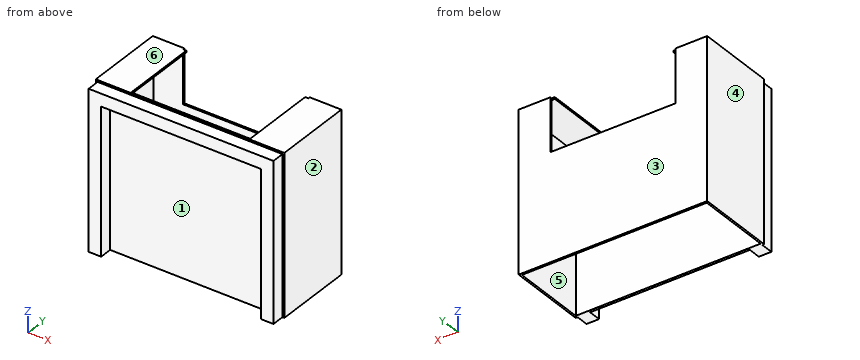
from build123d import *

# Parameters (mm, degrees)
SKETCH_1_W          = 602.574462866
SKETCH_1_H          = 504.761774505
EXTRUDE_1_DEPTH     = 8
SKETCH_2_W          = 6
SKETCH_2_H          = 504.761774505
EXTRUDE_2_DEPTH     = 240
SKETCH_3_W          = 602.574462866
SKETCH_3_H          = 504.761774505
EXTRUDE_3_DEPTH     = 6
SKETCH_5_W          = 602.574462866
SKETCH_5_H          = 254
EXTRUDE_4_DEPTH     = 6
SKETCH_4_W          = 400
SKETCH_4_H          = 170
CUT_EXTRUDE_4_DEPTH = 6
SKETCH_9_W          = 380
SKETCH_9_H          = 245
CUT_EXTRUDE_5_DEPTH = 6
EXTRUDE_8_DEPTH     = 40


with BuildPart() as part:
    # Эскиз1 → Бобышка-Вытянуть1 (new body)
    with BuildSketch(Plane(origin=(0, 0, 0), x_dir=(1, 0, 0), z_dir=(0, 1, 0))):
        with Locations((300, -321.529892077)):
            Rectangle(SKETCH_1_W, SKETCH_1_H)
    extrude(amount=EXTRUDE_1_DEPTH)

    # Эскиз2 → Бобышка-Вытянуть2 (add)
    with BuildSketch(Plane(origin=(0, 8, 0), x_dir=(1, 0, 0), z_dir=(0, 1, 0))):
        with Locations((1.712768567, -321.529892077)):
            Rectangle(SKETCH_2_W, SKETCH_2_H)
        with Locations((598.287231433, -321.529892077)):
            Rectangle(SKETCH_2_W, SKETCH_2_H)
    extrude(amount=EXTRUDE_2_DEPTH)

    # Эскиз3 → Бобышка-Вытянуть3 (add)
    with BuildSketch(Plane(origin=(0, 248, 0), x_dir=(1, 0, 0), z_dir=(0, 1, 0))):
        with Locations((300, -321.529892077)):
            Rectangle(SKETCH_3_W, SKETCH_3_H)
    extrude(amount=EXTRUDE_3_DEPTH)

    # Эскиз5 → Бобышка-Вытянуть4 (add)
    with BuildSketch(Plane.XY.offset(573.910779329)):
        with Locations((300, 127)):
            Rectangle(SKETCH_5_W, SKETCH_5_H)
    extrude(amount=EXTRUDE_4_DEPTH)

    # Эскиз4 → Вырез-Вытянуть4 (cut)
    with BuildSketch(Plane(origin=(0, 254, 0), x_dir=(1, 0, 0), z_dir=(0, 1, 0))):
        with Locations((300, -494.910779329)):
            Rectangle(SKETCH_4_W, SKETCH_4_H)
    extrude(amount=-CUT_EXTRUDE_4_DEPTH, mode=Mode.SUBTRACT)

    # Эскиз9 → Вырез-Вытянуть5 (cut)
    with BuildSketch(Plane.XY.offset(579.910779329)):
        with Locations((300, 125.5)):
            Rectangle(SKETCH_9_W, SKETCH_9_H)
    extrude(amount=-CUT_EXTRUDE_5_DEPTH, mode=Mode.SUBTRACT)

    # Эскиз12 → Бобышка-Вытянуть8 (add)
    with BuildSketch(Plane.XZ):
        Polygon((4.712768567, 573.910779329), (595.287231433, 573.910779329), (595.287231433, 69.149004824), (555.287231433, 69.149004824), (555.287231433, 533.910779329), (44.712768567, 533.910779329), (44.712768567, 69.149004824), (4.712768567, 69.149004824), align=None)
    extrude(amount=EXTRUDE_8_DEPTH)


solid = part.part
Source: CAD feature listing. Evaluate the final solid. Frame: model axes, mm. Face numbers are marked on the shaded views. A direction names the side the tool comes from. Round coordinates to 2 decimals unless told otherwise and drop trailing zeros. Loops run counter-clockwise (first coordinate to the right, second up) from the corner with the lowest first, then second, coordinate; pieces in that order, holes last. Notation, with made-up numbers: (-6, 34) -> (45, 34) arc R19 ccw to (45, 65) -> close; hole circle Ø8 at (66, 4.25). An arc over 180 degrees is marked (long way). Answer as a JSON object with one key per item and string values. Group by question number.
Q1. Section query A-A (y = 205.5). Output: boundary loops of the cut face in (x, z).
Q2. Mould query, pull axis X, two halves, no side actions, for the marked faces 1, 2, 3 and 4. Classes: pulls with the +X half, pulls with the -X half, needs draft (parallel to the pull), parting line crosses it, or undercut.
Q3. Section query D-D (z = 439.5). Output: boundary loops of the cut face in (x, y).
Q4. Section query C-C (z = 113.5). Output: boundary loops of the cut face in (x, y).
Q5. Ray query, line 1 (Y direction, x = 463.5, z = 148.5); line 2 (X direction, y = 133, z = 264); line 3 (Y direction, x = 29, z = 376). Return the intervals inside material, ascending. Write a range as from..to.
Q6. Section query B-B (x = 121). Output: boundary loops of the cut face in (y, z).
Q7. Contact query for flat-ended pins moving along their axis: P1, Ø12, axis at x = 214, y = -29, coming from the +Z side; P2, Ø20, axis at y = -12.5, z = 247, coming from the +X side; P3, Ø5, axis at x = 220, y = 251.5, coming from the +Z side. Output: stop coordinate, or through.
Q8. Access query for the marked faces 5 and 6. Directions: +Z, -Z, +X, -X, +Y, -Y. A direction counts if a zero-diameter tool reaches every point of the face in a straight line with its end or side. Return the directions, or none.
Completed:
{
 "1": {"outline": "(-1.29, 69.15) -> (4.71, 69.15) -> (4.71, 573.91) -> (110, 573.91) -> (110, 579.91) -> (-1.29, 579.91) -> close; (490, 573.91) -> (595.29, 573.91) -> (595.29, 69.15) -> (601.29, 69.15) -> (601.29, 579.91) -> (490, 579.91) -> close"},
 "2": {"face 1": "undercut", "face 2": "pulls with the +X half", "face 3": "needs draft", "face 4": "pulls with the -X half"},
 "3": {"outline": "(-1.29, 0) -> (4.71, 0) -> (4.71, -40) -> (44.71, -40) -> (44.71, 0) -> (555.29, 0) -> (555.29, -40) -> (595.29, -40) -> (595.29, 0) -> (601.29, 0) -> (601.29, 254) -> (500, 254) -> (500, 248) -> (595.29, 248) -> (595.29, 8) -> (4.71, 8) -> (4.71, 248) -> (100, 248) -> (100, 254) -> (-1.29, 254) -> close"},
 "4": {"outline": "(-1.29, 0) -> (4.71, 0) -> (4.71, -40) -> (44.71, -40) -> (44.71, 0) -> (555.29, 0) -> (555.29, -40) -> (595.29, -40) -> (595.29, 0) -> (601.29, 0) -> (601.29, 254) -> (-1.29, 254) -> close; hole (4.71, 8) -> (595.29, 8) -> (595.29, 248) -> (4.71, 248) -> close"},
 "5": {"line 1": "0..8, 248..254", "line 2": "-1.29..4.71, 595.29..601.29", "line 3": "-40..8, 248..254"},
 "6": {"outline": "(-40, 533.91) -> (0, 533.91) -> (0, 69.15) -> (8, 69.15) -> (8, 573.91) -> (3, 573.91) -> (3, 579.91) -> (0, 579.91) -> (0, 573.91) -> (-40, 573.91) -> close; (248, 69.15) -> (254, 69.15) -> (254, 409.91) -> (248, 409.91) -> close"},
 "7": {"P1": "z = 573.91", "P2": "x = 595.29", "P3": "z = 409.91"},
 "8": {"face 5": "-Z", "face 6": "+Z, +X, -X, +Y, -Y"}
}
